```python
from build123d import *

# Parameters (mm, degrees)
SKETCH1_R               = 1
BOSS_EXTRUDE1_DEPTH     = 2
SKETCH4_R               = 1
BOSS_EXTRUDE2_DEPTH     = 11
SKETCH11_W              = 0.548452347
SKETCH11_H              = 0.731269796
BOSS_EXTRUDE3_DEPTH     = 1
SKETCH12_W              = 2.985960681
SKETCH12_H              = 2.799338139
BOSS_EXTRUDE4_DEPTH     = 3
SKETCH15_W              = 5
SKETCH15_H              = 2
BOSS_EXTRUDE5_DEPTH     = 86.79
CUT_EXTRUDE4_DEPTH      = 87.918088451
CUT_EXTRUDE4_DEPTH_BACK = 87.918088451
CUT_EXTRUDE5_DEPTH      = 88.033063258
CUT_EXTRUDE5_DEPTH_BACK = 88.033063258
SKETCH19_R              = 1.05
CUT_EXTRUDE7_DEPTH      = 87.918088451
CUT_EXTRUDE7_DEPTH_BACK = 87.918088451


with BuildPart() as part:
    # Sketch1 → Boss-Extrude1 (new body)
    with BuildSketch(Plane(origin=(0, 0, 0), x_dir=(1, 0, 0), z_dir=(0, 1, 0))):
        with BuildLine():
            Line((-10, 2.5), (0, 2.5))
            Line((0, 2.5), (0, -2.5))
            Line((0, -2.5), (-10, -2.5))
            ThreePointArc((-10, -2.5), (-12.5, 0), (-10, 2.5))
        make_face()
        with Locations(Location((-10, 0, 0), (0, 0, 270))):
            Circle(SKETCH1_R, mode=Mode.SUBTRACT)
    extrude(amount=BOSS_EXTRUDE1_DEPTH)

    # Sketch4 → Boss-Extrude2 (add)
    with BuildSketch(Plane(origin=(0, 0, 0), x_dir=(0, 0, -1), z_dir=(1, 0, 0))):
        with Locations(Location((0, 1, 0), (0, 0, 270))):
            Circle(SKETCH4_R)
    extrude(amount=BOSS_EXTRUDE2_DEPTH)

    # Sketch11 → Boss-Extrude3 (add)
    with BuildSketch(Plane.XZ):
        with Locations((-7.723091918, 0.104467114)):
            Rectangle(SKETCH11_W, SKETCH11_H)
    extrude(amount=BOSS_EXTRUDE3_DEPTH)

    # Sketch12 → Boss-Extrude4 (add)
    with BuildSketch(Plane.XZ.offset(1)):
        with Locations((-6.985405351, -0.467965971)):
            Rectangle(SKETCH12_W, SKETCH12_H)
    extrude(amount=BOSS_EXTRUDE4_DEPTH)

    # Sketch15 → Boss-Extrude5 (add)
    with BuildSketch(Plane(origin=(0, 0, 0), x_dir=(0, 0, -1), z_dir=(1, 0, 0))):
        with Locations((0, 1)):
            Rectangle(SKETCH15_W, SKETCH15_H)
    extrude(amount=-BOSS_EXTRUDE5_DEPTH)

    # Sketch16 → Cut-Extrude4 (cut, two sides: drawn at the far end of the back side and taken through both)
    with BuildSketch(Plane.XZ.offset(-CUT_EXTRUDE4_DEPTH_BACK)):
        with BuildLine():
            ThreePointArc((-84.29, -2.5), (-86.057766953, -1.767766953), (-86.79, 0))
            Line((-86.79, 0), (-86.79, -2.5))
            Line((-86.79, -2.5), (-84.29, -2.5))
        make_face()
    extrude(amount=CUT_EXTRUDE4_DEPTH + CUT_EXTRUDE4_DEPTH_BACK, mode=Mode.SUBTRACT)

    # Sketch19 → Cut-Extrude5 (cut, two sides: drawn at the far end of the back side and taken through both)
    with BuildSketch(Plane(origin=(0, 2, 0), x_dir=(1, 0, 0), z_dir=(0, 1, 0)).offset(-CUT_EXTRUDE5_DEPTH_BACK)):
        with Locations(Location((-84.29, 0, 0), (0, 0, 270))):
            Circle(SKETCH19_R)
    extrude(amount=CUT_EXTRUDE5_DEPTH + CUT_EXTRUDE5_DEPTH_BACK, mode=Mode.SUBTRACT)

    # Sketch16_4 → Cut-Extrude7 (cut, two sides: drawn at the far end of the back side and taken through both)
    with BuildSketch(Plane.XZ.offset(-CUT_EXTRUDE7_DEPTH_BACK)):
        with BuildLine():
            Line((-86.79, 2.5), (-86.79, 0))
            ThreePointArc((-86.79, 0), (-86.057766953, 1.767766953), (-84.29, 2.5))
            Line((-84.29, 2.5), (-86.79, 2.5))
        make_face()
    extrude(amount=CUT_EXTRUDE7_DEPTH + CUT_EXTRUDE7_DEPTH_BACK, mode=Mode.SUBTRACT)

    # Sketch22 → Revolve2 (revolve)
    with BuildSketch(Plane(origin=(0, 1, 0), x_dir=(-1, 0, 0), z_dir=(0, -1, 0))):
        with BuildLine():
            ThreePointArc((-7.5, 0), (-10, -2.5), (-12.5, 0))
            Line((-12.5, 0), (-7.5, 0))
        make_face()
    revolve(axis=Axis((12.5, 1, 0), (-1, 0, 0)))


solid = part.part
```
For this review, take the finished solid that the model builds, in its own axes (mm). A direction names the side the tool comes from. Coordinates: 2 decimals unless noted, no trailing zeros. Write each loop counter-clockwise with the first axis right and the second up, starting at its lowest first coordinate (ties: lowest second). Pieces come first, ordered by that corner, then holes.
(1) Tool access review of faces 1 (the face through (-43, 1, -2.5)), 2 (the face through (-8.478, -2, 0)), 3 (the face through (-43, 2, 0)), 4 (the face through (4, 1, 1)): name each direction out of +Z, -Z, +X, -X, +Y, -Y from which nothing blocks a thin tool from reaching the whole face with its end or side.
(2) Wall thickness on probe 1 along X at (y, z) = (1.3, 0); probe 2 along Z at (x, y) = (-84.29, 1); probe 3 along Y at (x, z) = (-9.5, -1.95): over which ranges is each line inside the solid? List them lowest first.
(3) Add section A-A on y = 1. Give the boundary of the cut face in (x, z).
(4) Add section B-B on x = 4. Give the boundary of the cut face in (y, z), then the cut area to 3 significant figures.
(5) Add section C-C on x = -13. Give the boundary of the cut face in (y, z), then the cut area to 3 significant figures.
(6) For pin 1 Ø3 at (y, z) = (-2.5, -1) entering from -X; pin 2 Ø1.5 at (x, y) = (-7.5, -2.5) entering from -Z; pin 3 Ø2 at (x, z) = (-7.5, 0) entering from +Y, all flat-tipped, find the tip position at first contact; note any pin that passes through.
(7) The part is to be moulded in two halves that separate along Y. For faces 5 (the face through (-7, -2, -1.868)), 6 (the face through (-7, -4, 0)), 7 (the face through (-7, -1, 0)), say which applies: +Y half, -Y half, draft (parallel to the pull), parting line (faces both ways), or undercut.
Answer sheet:
1. face 1: -Z, +X, -X, +Y, -Y
1. face 2: +Z, -Z, -X, -Y
1. face 3: +Z, -Z, -X, +Y
1. face 4: none
2. probe 1: x = -86.79 to -85.34, -83.24 to 12.48
2. probe 2: z = -2.5 to -1.05, 1.05 to 2.5
2. probe 3: y = 0 to 2
3. outline: (-84.29, -2.5) - (0, -2.5) - (0, -1) - (7.71, -1) arc R2.5 ccw (long way) to (7.71, 1) - (0, 1) - (0, 2.5) - (-84.29, 2.5) arc R2.5 ccw to start; hole circle Ø2.1 at (-84.29, 0)
4. outline: circle Ø2 at (1, 0)
4. area: 3.14 mm2
5. outline: (0, -2.5) - (2, -2.5) - (2, 2.5) - (0, 2.5) - close
5. area: 10.0 mm2
6. pin 1: stops at x = -8.48
6. pin 2: stops at z = -1.87
6. pin 3: stops at y = 2
7. face 5: draft
7. face 6: -Y half
7. face 7: undercut
